Verification items for the finished model (mm, model axes). A direction names the side the tool comes from. Give positions to 0.01 mm unless a question says otherwise; leave off trailing zeros. Order: outer loops, then holes, each group sorted by start corner. A loop starts at its lowest first (then second) coordinate and runs counter-clockwise, first axis right, second up. Notation, with made-up numbers: (68.25, -17) - (101.25, -17) arc R11 cw to (101.25, -5) - close; hole circle Ø3 at (75, -20). An arc over 180 degrees is marked (long way). Answer as a JSON object with one key per item and string values.
```python
from build123d import *

# Parameters (mm, degrees)
SKETCH1_W           = 24.8
SKETCH1_H           = 50.6
BOSS_EXTRUDE1_DEPTH = 2
BOSS_EXTRUDE2_DEPTH = 2
SKETCH3_W           = 10.61
SKETCH3_H           = 6.12
CUT_EXTRUDE1_DEPTH  = 3
FILLET1_R           = 5


with BuildPart() as part:
    # Sketch1 → Boss-Extrude1 (new body)
    with BuildSketch(Plane(origin=(0, 0, 0), x_dir=(1, 0, 0), z_dir=(0, 1, 0))):
        Rectangle(SKETCH1_W, SKETCH1_H)
    extrude(amount=BOSS_EXTRUDE1_DEPTH)

    # Sketch2 → Boss-Extrude2 (add)
    with BuildSketch(Plane(origin=(0, 2, 0), x_dir=(1, 0, 0), z_dir=(0, 1, 0))):
        Polygon((-7.4, 20.3), (7.4, 20.3), (7.4, -20.3), (4.5, -20.3), (4.5, -22.3), (9.4, -22.3), (9.4, 22.3), (-9.4, 22.3), (-9.4, -22.3), (-4.5, -22.3), (-4.5, -20.3), (-7.4, -20.3), align=None)
    extrude(amount=BOSS_EXTRUDE2_DEPTH)

    # Sketch3 → Cut-Extrude1 (cut, through all)
    with BuildSketch(Plane(origin=(0, 2, 0), x_dir=(1, 0, 0), z_dir=(0, 1, 0))):
        with Locations((0, 15.94)):
            Rectangle(SKETCH3_W, SKETCH3_H)
    extrude(amount=-CUT_EXTRUDE1_DEPTH, mode=Mode.SUBTRACT)

    # Fillet1
    fillet1_edges = [part.edges().sort_by_distance(p)[0] for p in [
        (12.4, 1, -25.3),
        (12.4, 1, 25.3),
        (-12.4, 1, 25.3),
        (-12.4, 1, -25.3),
    ]]
    fillet(fillet1_edges, radius=FILLET1_R)


solid = part.part
```
(1) Access from +Z, -Z, +X, -X, +Y, -Y to the whole of each face (thin tool, end or side, straight path). Record for faces 1 (the flat face through (0, 3, -22.3)), 2 (the flat face through (-7.4, 3, 0)), 3 (the flat face through (-7, 3, 22.3)), 4 (the flat face through (-4.5, 3, 21)).
Computed values:
{"face 1": "-Z, +X, -X, +Y", "face 2": "+Y", "face 3": "+Z, +X, -X, +Y", "face 4": "+Z, +Y"}
(2) Section check D-D (y = 2.85). Record the cut outline in (x, z), then the cut area to 3 significant figures.
Computed values:
{"outline": "(-9.4, -22.3) - (9.4, -22.3) - (9.4, 22.3) - (4.5, 22.3) - (4.5, 20.3) - (7.4, 20.3) - (7.4, -20.3) - (-7.4, -20.3) - (-7.4, 20.3) - (-4.5, 20.3) - (-4.5, 22.3) - (-9.4, 22.3) - close", "area": "220 mm²"}
(3) Section check A-A (x = 0.75). Record the cut outline in (y, z), then the cut area to 3 significant figures.
Computed values:
{"outline": "(0, -25.3) - (2, -25.3) - (2, -22.3) - (4, -22.3) - (4, -20.3) - (2, -20.3) - (2, -19) - (0, -19) - close; (0, -12.88) - (2, -12.88) - (2, 25.3) - (0, 25.3) - close", "area": "93.0 mm²"}
(4) Gauge pin test, flat ends, axial feed: pin 1 Ø2 at (y, z) = (3.5, -15) entering from -X; pin 2 Ø8 at (x, z) = (-2, -10.5) entering from +Y; pin 3 Ø1.6 at (y, z) = (3, 21) entering from +X. Record the tip position at first contact, or that the pin passes through.
Computed values:
{"pin 1": "stops at x = -9.4", "pin 2": "stops at y = 2", "pin 3": "stops at x = 9.4"}
(5) Release check for a two-part mould opening along X. For faces 5 (the flat face through (-12.4, 1, 0)), 6 (the flat face through (-8, 4, 2)), 7 (the flat face through (7.4, 3, 0)) record: pulls with the +X half, pulls with the -X half, needs draft (parallel to the pull), parting line crosses it, or undercut.
Computed values:
{"face 5": "pulls with the -X half", "face 6": "needs draft", "face 7": "undercut"}
(6) Section check B-B (y = 0.8). Record the cut outline in (x, z) (3 decimals).
Computed values:
{"outline": "(-12.4, -20.3) arc R5 ccw to (-7.4, -25.3) - (7.4, -25.3) arc R5 ccw to (12.4, -20.3) - (12.4, 20.3) arc R5 ccw to (7.4, 25.3) - (-7.4, 25.3) arc R5 ccw to (-12.4, 20.3) - close; hole (-5.305, -19) - (5.305, -19) - (5.305, -12.88) - (-5.305, -12.88) - close"}
(7) Material ranges on line 1 along X through (y, z) = (2.9, 0.5); line 2 along X through (y, z) = (3.05, 20.5); line 3 along Z through (x, y) = (-2.25, 1.5), recorded low to high. Write a range as [from, to].
Computed values:
{"line 1": "x = [-9.4, -7.4], [7.4, 9.4]", "line 2": "x = [-9.4, -4.5], [4.5, 9.4]", "line 3": "z = [-25.3, -19], [-12.88, 25.3]"}
(8) Section check C-C (z = -16.5). Record the cut outline in (x, y) (3 decimals), then the cut area to 3 significant figures.
Computed values:
{"outline": "(-12.4, 0) - (-5.305, 0) - (-5.305, 2) - (-7.4, 2) - (-7.4, 4) - (-9.4, 4) - (-9.4, 2) - (-12.4, 2) - close; (5.305, 0) - (12.4, 0) - (12.4, 2) - (9.4, 2) - (9.4, 4) - (7.4, 4) - (7.4, 2) - (5.305, 2) - close", "area": "36.4 mm²"}
